Study the drawing (mm; zero at the part's minimum x, y, z) and answer. Round coordinates to 2 decimals unless told otherwise and drop trailing zeros. Order: outer loops, then holes, each group sorted by start corner. A loop starts at its lowest first (then second) coordinate and runs counter-clockwise, first axis right, second up. Notation, with made-up numbers: (86.5, 64.25) - (93.5, 64.25) arc R25 ccw to (93.5, 84.25) - close; hole circle Ø7 at (43.25, 52.25). An arc over 180 degrees is marked (long way). Put each result on its own line as item: value.
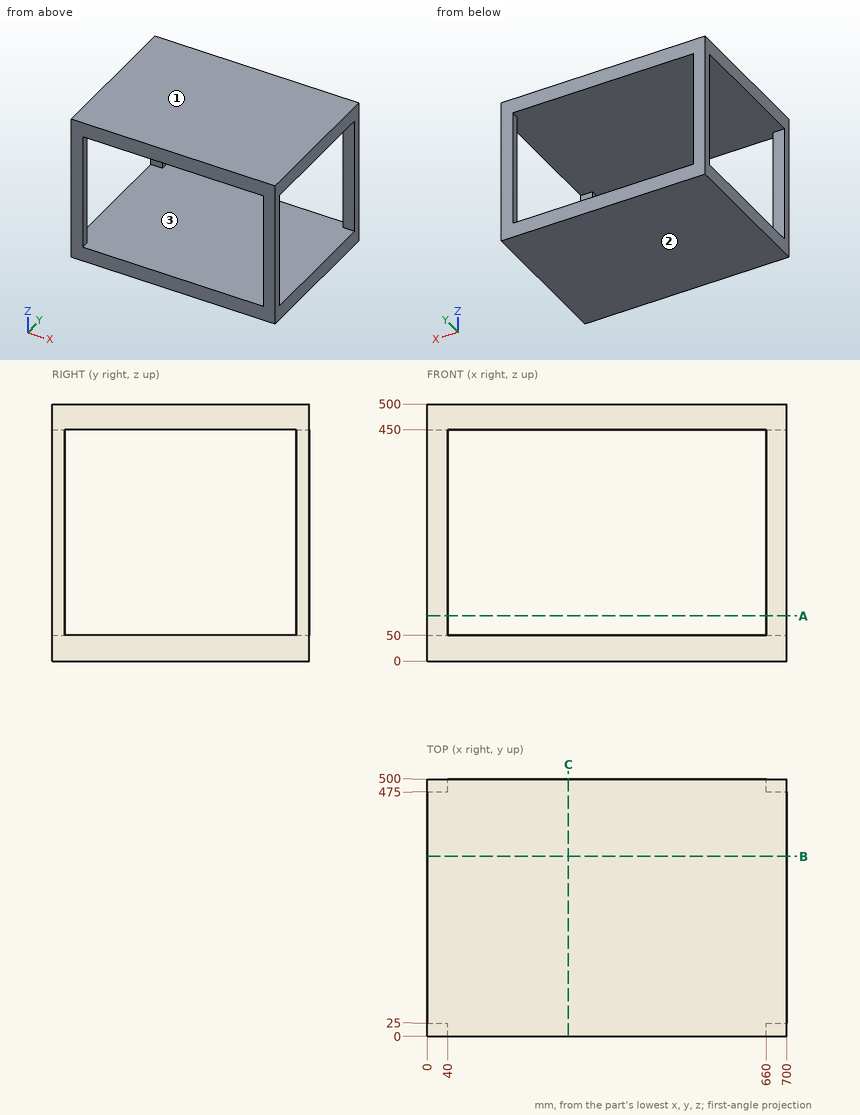
1) A cutting plane is placed at B-B on y = 349.5. Write down the section's boundary in (x, z).
Findings below:
outline: (0, 0) - (700, 0) - (700, 50) - (0, 50) - close; (0, 450) - (700, 450) - (700, 500) - (0, 500) - close
2) A cutting plane is placed at C-C on x = 275. Write down the section's boundary in (y, z), then the cut area to 3 significant figures.
Findings below:
outline: (0, 0) - (500, 0) - (500, 50) - (0, 50) - close; (0, 450) - (500, 450) - (500, 500) - (0, 500) - close
area: 50,000 mm2
3) Straight lines are drawn through the part: L1, parallel to Z at x = 210.5, y = 277; L2, parallel to Y at x = 660.5, z = 243; L3, parallel to X at y = 22.5, z = 65. For each, find the intervals that lie inside material, in ascending order. Write a range as from..to.
Findings below:
L1: z = 0..50, 450..500
L2: y = 0..25, 475..500
L3: x = 0..40, 660..700
4) For a pull along Z with two mould halves and no side action, classify the marked faces 1, 2 and 3 as pulls with the +Z half, pulls with the -Z half, needs draft (parallel to the pull), parting line crosses it, or undercut.
Findings below:
face 1: pulls with the +Z half
face 2: pulls with the -Z half
face 3: undercut
5) A cutting plane is placed at A-A on z = 88. Write down the section's boundary in (x, y), then the cut area to 3 significant figures.
Findings below:
outline: (0, 0) - (40, 0) - (40, 25) - (0, 25) - close; (0, 475) - (40, 475) - (40, 500) - (0, 500) - close; (660, 0) - (700, 0) - (700, 25) - (660, 25) - close; (660, 475) - (700, 475) - (700, 500) - (660, 500) - close
area: 4,000 mm2
